Autodesk Inventor part; units mm, degrees
ref_plane "YZ Plane" through (0, 0, 0) normal (1, 0, 0) x (0, 1, 0)
ref_plane "XZ Plane" through (0, 0, 0) normal (0, 1, 0) x (-1, 0, 0)
ref_plane "XY Plane" through (0, 0, 0) normal (0, 0, 1) x (1, 0, 0)
sketch "Sketch1" plane through (0, 0, 0) normal (0, 1, 0) x (-1, 0, 0)
  circle A0 centre (0, 0) radius 200
  circle A1 centre (0, 0) radius 220
  line L0 (220, 0) -> (200, 0)
  line L1 (-220, 0) -> (-200, 0)
  line L2 (0, 0) -> (-200, 0) construction
  line L3 (0, 200) -> (0, 0) construction
  line L4 (0, 220) -> (0, 200)
  line L5 (-200, 0) -> (-220, 0)
  line L6 (-204, 7) -> (-216, 7)
  line L7 (-216, 7) -> (-213.4522, 0)
  line L8 (-204, 7) -> (-206.5478, 0)
  line L9 (-210, 0) -> (-210, 7) construction
  line L10 (-203.4647, 58.0945) -> (-193.2038, 86.2852)
  line L11 (-193.2038, 86.2852) -> (-190.1968, 85.1907)
  line L12 (-190.1968, 85.1907) -> (-200.4577, 57)
  line L13 (-200.4577, 57) -> (-203.4647, 58.0945)
  line L14 (-203.4647, 58.0945) -> (-190.1968, 85.1907) construction
  line L15 (-193.2038, 86.2852) -> (-200.4577, 57) construction
  circle A2 centre (0, 0) radius 210 construction
  line L16 (-7, -204) -> (0, -206.5478)
  line L17 (-7, -216) -> (0, -213.4522)
  line L18 (-7, -204) -> (-7, -216)
  line L19 (204, -7) -> (206.5478, 0)
  line L20 (216, -7) -> (213.4522, 0)
  line L21 (204, -7) -> (216, -7)
  line L22 (7, 204) -> (0, 206.5478)
  line L23 (7, 216) -> (0, 213.4522)
  line L24 (7, 204) -> (7, 216)
  line L25 (-205.2528, -51.421) -> (-210.462, -21.8768)
  line L26 (-202.1014, -50.8654) -> (-205.2528, -51.421)
  line L27 (-207.3106, -21.3211) -> (-202.1014, -50.8654)
  line L28 (-210.462, -21.8768) -> (-207.3106, -21.3211)
  line L29 (-152.0436, -147.1583) -> (-171.3271, -124.1768)
  line L30 (-149.5923, -145.1014) -> (-152.0436, -147.1583)
  line L31 (-168.8757, -122.1199) -> (-149.5923, -145.1014)
  line L32 (-171.3271, -124.1768) -> (-168.8757, -122.1199)
  line L33 (-58.0945, -203.4647) -> (-86.2852, -193.2038)
  line L34 (-57, -200.4577) -> (-58.0945, -203.4647)
  line L35 (-85.1907, -190.1968) -> (-57, -200.4577)
  line L36 (-86.2852, -193.2038) -> (-85.1907, -190.1968)
  line L37 (51.421, -205.2528) -> (21.8768, -210.462)
  line L38 (50.8654, -202.1014) -> (51.421, -205.2528)
  line L39 (21.3211, -207.3106) -> (50.8654, -202.1014)
  line L40 (21.8768, -210.462) -> (21.3211, -207.3106)
  line L41 (147.1583, -152.0436) -> (124.1768, -171.3271)
  line L42 (145.1014, -149.5923) -> (147.1583, -152.0436)
  line L43 (122.1199, -168.8757) -> (145.1014, -149.5923)
  line L44 (124.1768, -171.3271) -> (122.1199, -168.8757)
  line L45 (203.4647, -58.0945) -> (193.2038, -86.2852)
  line L46 (200.4577, -57) -> (203.4647, -58.0945)
  line L47 (190.1968, -85.1907) -> (200.4577, -57)
  line L48 (193.2038, -86.2852) -> (190.1968, -85.1907)
  line L49 (205.2528, 51.421) -> (210.462, 21.8768)
  line L50 (202.1014, 50.8654) -> (205.2528, 51.421)
  line L51 (207.3106, 21.3211) -> (202.1014, 50.8654)
  line L52 (210.462, 21.8768) -> (207.3106, 21.3211)
  line L53 (152.0436, 147.1583) -> (171.3271, 124.1768)
  line L54 (149.5923, 145.1014) -> (152.0436, 147.1583)
  line L55 (168.8757, 122.1199) -> (149.5923, 145.1014)
  line L56 (171.3271, 124.1768) -> (168.8757, 122.1199)
  line L57 (58.0945, 203.4647) -> (86.2852, 193.2038)
  line L58 (57, 200.4577) -> (58.0945, 203.4647)
  line L59 (85.1907, 190.1968) -> (57, 200.4577)
  line L60 (86.2852, 193.2038) -> (85.1907, 190.1968)
  line L61 (-51.421, 205.2528) -> (-21.8768, 210.462)
  line L62 (-50.8654, 202.1014) -> (-51.421, 205.2528)
  line L63 (-21.3211, 207.3106) -> (-50.8654, 202.1014)
  line L64 (-21.8768, 210.462) -> (-21.3211, 207.3106)
  line L65 (-147.1583, 152.0436) -> (-124.1768, 171.3271)
  line L66 (-145.1014, 149.5923) -> (-147.1583, 152.0436)
  line L67 (-122.1199, 168.8757) -> (-145.1014, 149.5923)
  line L68 (-124.1768, 171.3271) -> (-122.1199, 168.8757)
  point P0 (210, 0)
  point P1 (-210, 0)
  point P2 (-196.8307, 71.6426)
  point P3 (-40.1486, 206.1264)
  point P4 (-201.9612, 57.5472)
  point P5 (-191.7003, 85.7379)
  point P6 (-7, -210)
  point P7 (210, -7)
  point P8 (7, 210)
  point P9 (-203.6771, -51.1432)
  point P10 (-208.8863, -21.5989)
  point P11 (-150.818, -146.1299)
  point P12 (-170.1014, -123.1484)
  point P13 (-57.5472, -201.9612)
  point P14 (-85.7379, -191.7003)
  point P15 (51.1432, -203.6771)
  point P16 (21.5989, -208.8863)
  point P17 (146.1299, -150.818)
  point P18 (123.1484, -170.1014)
  point P19 (201.9612, -57.5472)
  point P20 (191.7003, -85.7379)
  point P21 (203.6771, 51.1432)
  point P22 (208.8863, 21.5989)
  point P23 (150.818, 146.1299)
  point P24 (170.1014, 123.1484)
  point P25 (57.5472, 201.9612)
  point P26 (85.7379, 191.7003)
  point P27 (-51.1432, 203.6771)
  point P28 (-21.5989, 208.8863)
  point P29 (-146.1299, 150.818)
  point P30 (-123.1484, 170.1014)
  point P31 (-206.5478, 0)
  point P32 (0, 206.5478)
  point P33 (0, 213.4522)
  dimension "d0" = 400
  dimension "d1" = 440
  dimension "d4" = 90
  dimension "d5" = 7
  dimension "d6" = 70
  dimension "d8" = 12
  dimension "d13" = 3.2
  dimension "d14" = 30
  dimension "d15" = 50
  dimension "d20" = 420
  dimension "d23" = 360
  dimension "d27" = 360
extrude "Extrusion1" add sketch "Sketch1" along normal blind 3 contours A0 L1 L8 L6 L7 A1 L4 | L4 L23 L24 L22
properties part number "R40_CM_CIRCULO"
Read the model definition and answer for the solid it produces. Units are mm, in the model's axes. A direction names the side the tool comes from. Give positions to 0.01 mm unless a question says otherwise; leave off trailing zeros. Write each loop counter-clockwise with the first axis right and the second up, starting at its lowest first coordinate (ties: lowest second). Pieces come first, ordered by that corner, then holes. Notation, with made-up numbers: (68, 16) -> (76, 16) arc R36 ccw to (76, 54) -> close; hole circle Ø3 at (25, 13.5). An arc over 180 degrees is marked (long way). Answer as a JSON object with one key per item and string values.
1) Section D-D on z = 49.5 is taken. Write down the section's boundary in (x, y), then the cut area to 3 significant figures.
Findings below:
{"outline": "(193.78, 0) -> (214.36, 0) -> (214.36, 3) -> (193.78, 3) -> close", "area": "61.7 mm^2"}
2) Straight lines are drawn through the part: probe 1 along Z at (x, y) = (39, 2); probe 2 along Z at (x, y) = (138, 1.6); probe 3 along X at (y, z) = (1.6, 64). For each, find the intervals that lie inside material, in ascending order. Write a range as from..to.
Findings below:
{"probe 1": "z = 196.16..204.19, 207.44..216.52", "probe 2": "z = 144.76..155.55, 159.73..171.34", "probe 3": "x = 189.48..197.91, 201.32..210.49"}
3) A tool of negligible diameter and unlimited length cuts with its end or side. For faces 5 (the flat face through (195.255, 1.479, 71.293)), 6 (the flat face through (141, 3, 143)), from which of +Z, -Z, +X, -X, +Y, -Y can it reach the whole face along a straight path? Write none if from no direction.
Findings below:
{"face 5": "+Y, -Y", "face 6": "+Z, -Z, +X, -X, +Y"}
4) A flat-ended cylindrical pin translates along its axis: pin 1 Ø0.9 at (x, y) = (208, 1) entering from -Z. Find the tip coordinate at first contact, or state that the pin passes through.
Findings below:
{"pin 1": "stops at z = 7"}
5) For a pull along Z with two mould halves and no side action, classify faces 1 (the flat face through (198.406, 1.479, 71.993)), 2 (the flat face through (141, 0, 143)), 3 (the cylindrical face through (142.968, 1.479, 139.858)), 4 (the cylindrical face through (157.265, 1.479, 153.844)) as pulls with the +Z half, pulls with the -Z half, needs draft (parallel to the pull), parting line crosses it, or undercut.
Findings below:
{"face 1": "undercut", "face 2": "needs draft", "face 3": "pulls with the -Z half", "face 4": "pulls with the +Z half"}
6) Section B-B on x = 28.5 is taken. Write down the section's boundary in (y, z), then the cut area to 3 significant figures.
Findings below:
{"outline": "(0, 197.96) -> (3, 197.96) -> (3, 206.04) -> (0, 206.04) -> close; (0, 209.29) -> (3, 209.29) -> (3, 218.15) -> (0, 218.15) -> close", "area": "50.8 mm^2"}
7) Section C-C on x = 137.5 is taken. Write down the section's boundary in (y, z), then the cut area to 3 significant figures.
Findings below:
{"outline": "(0, 145.24) -> (3, 145.24) -> (3, 155.97) -> (0, 155.97) -> close; (0, 160.15) -> (3, 160.15) -> (3, 171.74) -> (0, 171.74) -> close", "area": "67.0 mm^2"}
8) Section A-A on y = 1.05 is taken. Write down the section's boundary in (x, z).
Findings below:
{"outline": "(-7, 204) -> (0, 206.55) -> (0, 200) arc R200 cw to (200, 0) -> (206.55, 0) -> (204, 7) -> (216, 7) -> (213.45, 0) -> (220, 0) arc R220 ccw to (0, 220) -> (0, 213.45) -> (-7, 216) -> close; hole (21.32, 207.31) -> (50.87, 202.1) -> (51.42, 205.25) -> (21.88, 210.46) -> close; hole (122.12, 168.88) -> (145.1, 149.59) -> (147.16, 152.04) -> (124.18, 171.33) -> close; hole (190.2, 85.19) -> (200.46, 57) -> (203.46, 58.09) -> (193.2, 86.29) -> close"}
